Geometry check sheet. Reference: the model listing, model coordinates, mm. A direction names the side the tool comes from. Coordinates: 2 decimals unless noted, no trailing zeros. Write each loop counter-clockwise with the first axis right and the second up, starting at its lowest first coordinate (ties: lowest second). Pieces come first, ordered by that corner, then holes. Notation, with made-up numbers: (51.5, 61) -> (59.5, 61) arc R21 cw to (59.5, 66) -> close; hole circle Ø5 at (18, -22.75). An arc over 180 degrees is marked (long way). One line per question, with ' | ' between items.
Autodesk Inventor part; units mm, degrees
ref_plane "YZ Plane" through (0, 0, 0) normal (1, 0, 0) x (0, 1, 0)
ref_plane "XZ Plane" through (0, 0, 0) normal (0, 1, 0) x (-1, 0, 0)
ref_plane "XY Plane" through (0, 0, 0) normal (0, 0, 1) x (1, 0, 0)
sketch "Sketch1" plane through (0, 0, 0) normal (1, 0, 0) x (0, 1, 0)
  line L0 (81.2, 2.1737) -> (83.2, 2.1737)
  line L1 (83.2, 2.1737) -> (83.2, 4.1737)
  line L2 (83.2, 4.1737) -> (87.2, 4.1737)
  line L3 (87.2, 4.1737) -> (87.2, 2.1737)
  line L4 (87.2, 2.1737) -> (90.2, 2.1737)
  line L5 (90.2, 2.1737) -> (90.2, 7.1737)
  arc A0 (90.2, 11.1737) -> (90.2, 7.1737) centre (90.2, 9.1737) ccw
  line L6 (90.2, 11.1737) -> (90.2, 16.1737)
  line L7 (90.2, 16.1737) -> (92.2, 16.1737)
  line L8 (92.2, 16.1737) -> (92.2, 16.1737)
  line L9 (92.2, 16.1737) -> (112.2, 16.1737)
  line L10 (112.2, 16.1737) -> (112.2, -5.8263)
  line L11 (112.2, -5.8263) -> (81.2, -5.8263)
  line L12 (81.2, -5.8263) -> (81.2, 2.1737)
  line L13 (90.2, 11.1737) -> (90.2, 7.1737) construction
  line L14 (0, -10.2263) -> (0, 20.5737)
  point P0 (0, 0)
  dimension "d0" = 4
  dimension "d1" = 9
  dimension "d2" = 3
  dimension "d3" = 2
  dimension "d4" = 5
  dimension "d5" = 4
  dimension "d6" = 90.2
  dimension "d8" = 20
  dimension "d9" = 2
  dimension "d21" = 81.2
  dimension "d22" = 8
  dimension "d23" = 14
  dimension "d25" = 22
  dimension "d40" = 0
revolve "Revolution1" add sketch "Sketch1" angle 45 mid plane about axis through (0, 0, -10) along (0, 0, 1)
chamfer "Chamfer2" distance 1 angle 45 4 edges at (0, 83.2, 4.1737) (0, 87.2, 4.1737) (0, 81.2, 2.1737) (0, 90.2, 16.1737)
chamfer "Chamfer3" distance 2 angle 45 2 edges at (0, 112.2, -5.8263) (0, 112.2, 16.1737)
sketch "Sketch5" plane through (0, 0, 16.1737) normal (0, 0, 1) x (1, 0, 0)
  circle A0 centre (26.6584, 99.4904) radius 5.25
  circle A1 centre (-26.6584, 99.4904) radius 5.25
  arc A2 (-1.1976, 102.993) -> (-50.3773, 89.8395) centre (0, 0) ccw construction
  line L0 (0, 0) -> (-26.6584, 99.4904) construction
  line L1 (0, -22.44) -> (0, 134.64) construction
  dimension "d41" = 103
  dimension "d42" = 10.5
  dimension "d43" = 15
extrude "Extrusion4" cut sketch "Sketch5" against normal through all
properties part number "prueba_clamp_iso160"
1. Cross-section at B-B on z = 12.5. Record the boundary of the cut face in (x, y).
Worked answers:
outline: (-42.94, 103.66) -> (-34.52, 83.33) arc R90.2 cw to (34.52, 83.33) -> (42.94, 103.66) arc R112.2 ccw to start; hole circle Ø10.5 at (-26.66, 99.49); hole circle Ø10.5 at (26.66, 99.49)
2. Material ranges on line 1 (Z direction, x = -34, y = 83.5); line 2 (Z direction, x = 1, y = 83); line 3 (Z direction, x = -8.5, y = 88.5), recorded low to high. Write a range as from..to.
Worked answers:
line 1: -5.83..2.17, 7.17..11.17 | line 2: -5.83..2.17 | line 3: -5.83..2.17, 7.65..10.7
3. Tool access check on faces 4 (the face through (-27.796, 94.365, 5.328)), 5 (the face through (-1, 88, 2.174)), 6 (the face through (-0.6, 84.4, 4.174)), 7 (the face through (-0.5, 87.2, 2.7)), 8 (the face through (-1, 100, 16.174)). Record the directions out of +Z, -Z, +X, -X, +Y, -Y that give a thin tool (end or side, any length) a straight path to the whole face; none if there is none.
Worked answers:
face 4: +Z, -Z | face 5: none | face 6: +Z, -Y | face 7: +Z | face 8: +Z, +X, -X, +Y, -Y
4. Cross-section at C-C on z = 9. Record the boundary of the cut face in (x, y).
Worked answers:
outline: (-42.94, 103.66) -> (-33.76, 81.49) arc R88.21 cw to (33.76, 81.49) -> (42.94, 103.66) arc R112.2 ccw to start; hole circle Ø10.5 at (-26.66, 99.49); hole circle Ø10.5 at (26.66, 99.49)
5. Mould release check, pull along Z, two halves, no side actions. Record for faces 1 (the face through (-0.6, 112.2, 5)), 2 (the face through (0.5, 90.2, 4.7)), 3 (the face through (0.458, 83.372, 3.347)): released by +Z, released by -Z, zero draft, split by the parting line, or undercut.
Worked answers:
face 1: zero draft | face 2: undercut | face 3: released by +Z
6. Cross-section at A-A on y = 96. Record the boundary of the cut face in (x, z).
Worked answers:
outline: (-39.76, -5.83) -> (-30.58, -5.83) -> (-30.58, 16.17) -> (-39.76, 16.17) -> close; (-22.74, -5.83) -> (22.74, -5.83) -> (22.74, 16.17) -> (-22.74, 16.17) -> close; (30.58, -5.83) -> (39.76, -5.83) -> (39.76, 16.17) -> (30.58, 16.17) -> close
7. Go/stop test with flat-tipped pins: P1, Ø8, axis at x = -5, z = 9.5, coming from the +Y side; P2, Ø5, axis at x = -7.5, z = 13.5, coming from the +Y side; P3, Ø6, axis at x = -25, z = 9, coming from the -Y side. Record where each tip stops, or that it passes through.
Worked answers:
P1: y = 112.2 | P2: y = 112.09 | P3: y = 83.64
